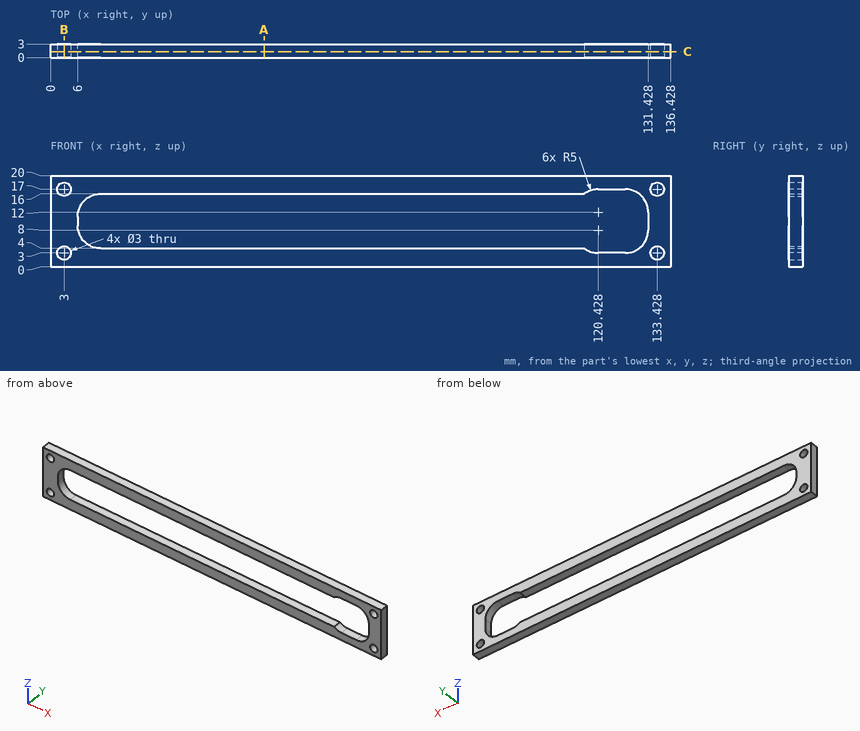
Check sheet for the drawn part. Datum: minimum x, y, z corner. Units: mm. Give positions to 0.01 mm unless a question says otherwise; leave off trailing zeros. Loops run counter-clockwise (first coordinate to the right, second up) from the corner with the lowest first, then second, coordinate; pieces in that order, holes last. Notation, with made-up numbers: M 21.5,88 L 78.5,88 A14 ccw 78.5,115 Z; hole C 86.25,-34.5 d9. An arc over 180 degrees is marked long. Answer as CSV lines item,"result".
Item 1: Scan lines: L1, parallel to Z at x = 3, y = 2; L2, parallel to Z at x = 63, y = 0.9; L3, parallel to X at y = 2.3, z = 8.5 (1 decimal). Record each from-to range of solid material in increasing order.
Reply:
L1,"0 to 1.5, 4.5 to 15.5, 18.5 to 20"
L2,"0 to 4, 16 to 20"
L3,"0 to 6, 131.4 to 136.4"
Item 2: Sectioned sample at C-C, the plane y = 1.3. Enter the section's corners in (x, z).
Reply:
outline,"M 0,0 L 136.43,0 L 136.43,20 L 0,20 Z; hole C 3,3 d3; hole C 3,17 d3; hole M 6,9 A5 ccw 11,4 L 117.43,4 A5 ccw 120.43,3 L 126.43,3 A5 ccw 131.43,8 L 131.43,12 A5 ccw 126.43,17 L 120.43,17 A5 ccw 117.43,16 L 11,16 A5 ccw 6,11 Z; hole C 133.43,3 d3; hole C 133.43,17 d3"
Item 3: Sectioned sample at A-A, the plane x = 47. Enter the section's corners in (y, z).
Reply:
outline,"M 0,0 L 3,0 L 3,4 L 0,4 Z; M 0,16 L 3,16 L 3,20 L 0,20 Z"
Item 4: Sectioned sample at B-B, the plane x = 3. Enter the section's corners in (y, z).
Reply:
outline,"M 0,0 L 3,0 L 3,1.5 L 0,1.5 Z; M 0,4.5 L 3,4.5 L 3,15.5 L 0,15.5 Z; M 0,18.5 L 3,18.5 L 3,20 L 0,20 Z"
